Print and shaded views of the part. All mm, measured from the part's lowest x, y and z. Round coordinates to 2 decimals unless told otherwise and drop trailing zeros. Write each loop counter-clockwise with the first axis right and the second up, starting at its lowest first coordinate (ties: lowest second). Pieces come first, ordered by that corner, then holes.
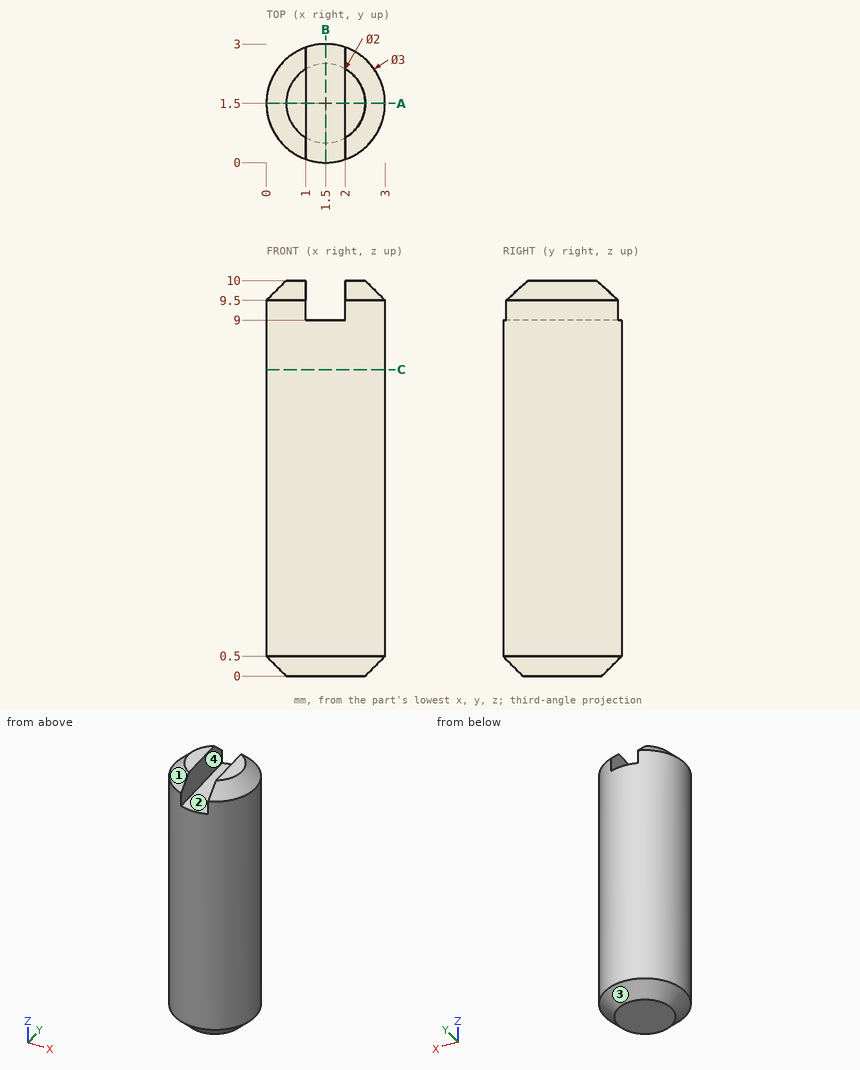
1) Slice it at C-C (z = 7.75). Write the cut outline in (x, y).
Results:
outline: circle Ø3 at (1.5, 1.5)
2) Pin check, flat tips, straight feed: pin 1 Ø0.5 at (x, y) = (1.5, 2) entering from +Z; pin 2 Ø0.5 at (y, z) = (2, 9.5) entering from -X; pin 3 Ø1.5 at (x, z) = (2.5, 7.5) entering from +Y. Stop position of each tip, or through.
Results:
pin 1: stops at z = 9
pin 2: stops at x = 0.02
pin 3: stops at y = 2.98
3) Slice it at B-B (x = 1.5). Write the cut outline in (y, z).
Results:
outline: (0, 0.5) - (0.5, 0) - (2.5, 0) - (3, 0.5) - (3, 9) - (0, 9) - close
4) Wall check: L1, parallel to Z at x = 1.4, y = 2.4; L2, parallel to X at y = 2.5, z = 9.25; L3, parallel to Y at x = 2.8, z = 8. Give the ranges that are in metal, low to high.
Results:
L1: z = 0 to 9
L2: x = 0.38 to 1, 2 to 2.62
L3: y = 0.75 to 2.25
5) Slice it at A-A (y = 1.5). Write the cut outline in (x, z).
Results:
outline: (0, 0.5) - (0.5, 0) - (2.5, 0) - (3, 0.5) - (3, 9.5) - (2.5, 10) - (2, 10) - (2, 9) - (1, 9) - (1, 10) - (0.5, 10) - (0, 9.5) - close
6) Mould opens along X. For the marked faces 1, 2, 3 and 4 say: released by +X, released by -X, zero draft, split by the parting line, or undercut.
Results:
face 1: released by -X
face 2: undercut
face 3: split by the parting line
face 4: undercut
